Autodesk Inventor part; units mm, degrees
ref_plane "YZ Plane" through (0, 0, 0) normal (1, 0, 0) x (0, 1, 0)
ref_plane "XZ Plane" through (0, 0, 0) normal (0, 1, 0) x (-1, 0, 0)
ref_plane "XY Plane" through (0, 0, 0) normal (0, 0, 1) x (1, 0, 0)
sketch "Sketch1" plane through (0, 0, 0) normal (0, 0, 1) x (1, 0, 0)
  line L0 (0, 17.78) -> (0, -17.78)
  line L1 (-34.29, 0) -> (27.94, 0)
  line L2 (-25.4, -12.7) -> (19.05, -12.7)
  line L3 (19.05, -12.7) -> (19.05, 12.7)
  line L4 (19.05, 12.7) -> (-25.4, 12.7)
  line L5 (-25.4, 12.7) -> (-25.4, -12.7)
  line L6 (-25.4, -12.7) -> (19.05, 12.7) construction
  line L7 (19.05, -12.7) -> (-25.4, 12.7) construction
  line L8 (-20.32, 0) -> (-10.82, 0) construction
  point P0 (0, 0)
  point P1 (-3.175, 0)
  point P2 (-15.57, 0)
  point P3 (0, 7.62)
  point P4 (0, -7.62)
  dimension "d0" = 44.45
  dimension "d1" = 25.4
  dimension "d3" = 19.05
  dimension "d4" = 9.5
  dimension "d5" = 0
  dimension "d6" = 7.62
  dimension "d7" = 7.62
  dimension "d25" = 5.08
extrude "Extrusion1" add sketch "Sketch1" along normal blind 5.842
hole "Hole1" at (-20.32, 0, 0) at (-10.82, 0, 0) direction (0, 0, 1) diameter 1.4986 end through all
hole "Hole2" at (0, 7.62, 0) at (0, -7.62, 0) direction (0, 0, 1) diameter 2.3622 end through all
fillet "Fillet1" radius 6.35 4 edges at (19.05, 12.7, 2.921) (-25.4, 12.7, 2.921) (-25.4, -12.7, 2.921) (19.05, -12.7, 2.921)
Work out the finished part from the listing and answer in its coordinate system (mm). Give positions to 0.01 mm unless a question says otherwise; leave off trailing zeros. Write each loop counter-clockwise with the first axis right and the second up, starting at its lowest first coordinate (ties: lowest second). Pieces come first, ordered by that corner, then holes. Notation, with made-up numbers: (66, -9.5) - (118, -9.5) arc R15 cw to (118, 18.5) - close; hole circle Ø1 at (27, 28). An arc over 180 degrees is marked (long way). Use one line per item in the form item = value.
1. Consider L1, parallel to X at y = 0, z = 4.2; L2, parallel to Y at x = 0, z = 4.4; L3, parallel to Y at x = -10.82, z = 2.9. Determine where each line is inside the solid, lowest interval first.
Filled in:
L1 = -25.4 to -21.07, -19.57 to -11.57, -10.07 to 19.05
L2 = -12.7 to -8.8, -6.44 to 6.44, 8.8 to 12.7
L3 = -12.7 to -0.75, 0.75 to 12.7
2. A cutting plane is placed at C-C (z = 2.2). Write down the section's boundary in (x, y), and give its area (3 significant figures).
Filled in:
outline = (-25.4, -6.35) arc R6.35 ccw to (-19.05, -12.7) - (12.7, -12.7) arc R6.35 ccw to (19.05, -6.35) - (19.05, 6.35) arc R6.35 ccw to (12.7, 12.7) - (-19.05, 12.7) arc R6.35 ccw to (-25.4, 6.35) - close; hole circle Ø1.5 at (-20.32, 0); hole circle Ø1.5 at (-10.82, 0); hole circle Ø2.36 at (0, -7.62); hole circle Ø2.36 at (0, 7.62)
area = 1,080 mm^2
3. Determine the mould class of faces 1 (the face through (-3, 0, 0)), 2 (the face through (-0.35, 8.75, 2.96)), 3 (the face through (17.24, 10.79, 2.96)) for opening direction Y: released by +Y, released by -Y, zero draft, split by the parting line, or undercut.
Filled in:
face_1 = zero draft
face_2 = undercut
face_3 = released by +Y
4. A cutting plane is placed at B-B (x = -10.82). Write down the section's boundary in (y, z), and give its area (3 significant figures).
Filled in:
outline = (-12.7, 0) - (-0.75, 0) - (-0.75, 5.84) - (-12.7, 5.84) - close; (0.75, 0) - (12.7, 0) - (12.7, 5.84) - (0.75, 5.84) - close
area = 140 mm^2
5. A cutting plane is placed at D-D (y = 7.62). Write down the section's boundary in (x, z), and give its area (3 significant figures).
Filled in:
outline = (-25.27, 0) - (-1.18, 0) - (-1.18, 5.84) - (-25.27, 5.84) - close; (1.18, 0) - (18.92, 0) - (18.92, 5.84) - (1.18, 5.84) - close
area = 244 mm^2
6. A cutting plane is placed at A-A (x = 0). Write down the section's boundary in (y, z).
Filled in:
outline = (-12.7, 0) - (-8.8, 0) - (-8.8, 5.84) - (-12.7, 5.84) - close; (-6.44, 0) - (6.44, 0) - (6.44, 5.84) - (-6.44, 5.84) - close; (8.8, 0) - (12.7, 0) - (12.7, 5.84) - (8.8, 5.84) - close
7. Each of these flat-tipped pins is pushed along its axis until it touches: pin 1 Ø1.9 at (x, y) = (-20.32, 0) entering from -Z; pin 2 Ø2 at (x, y) = (0, -7.62) entering from -Z. Where does it stop, or does it pass through?
Filled in:
pin_1 = 0
pin_2 = through
